Design review of the part built by this model. Coordinates are the model's own, in mm. Face numbers are marked on the shaded views. A direction names the side the tool comes from. Round coordinates to 2 decimals unless told otherwise and drop trailing zeros. Order: outer loops, then holes, each group sorted by start corner. A loop starts at its lowest first (then second) coordinate and runs counter-clockwise, first axis right, second up.
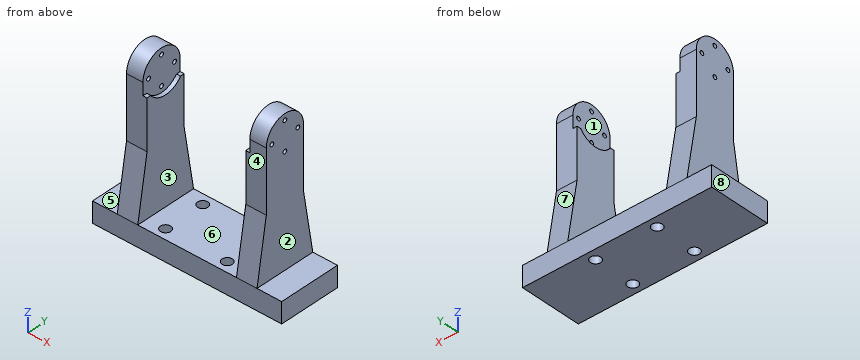
from build123d import *

# Parameters (mm, degrees)
SKETCH1_W           = 92
SKETCH1_H           = 30
BOSS_EXTRUDE1_DEPTH = 10
BOSS_EXTRUDE2_START = -12
BOSS_EXTRUDE2_DEPTH = 10
SKETCH3_R           = 1
CUT_EXTRUDE1_DEPTH  = 10
CUT_EXTRUDE2_DEPTH  = 2
SKETCH7_R           = 2.5
CUT_EXTRUDE3_DEPTH  = 10


with BuildPart() as part:
    # Sketch1 → Boss-Extrude1 (new body)
    with BuildSketch(Plane.XY):
        Rectangle(SKETCH1_W, SKETCH1_H)
    extrude(amount=BOSS_EXTRUDE1_DEPTH)

    # Sketch2 → Boss-Extrude2 (add)
    with BuildSketch(Plane(origin=(46, 0, 0), x_dir=(0, 0, -1), z_dir=(1, 0, 0)).offset(BOSS_EXTRUDE2_START)):
        with BuildLine():
            Line((-10, -15), (-10, 15))
            Line((-10, 15), (-40, 10))
            Line((-40, 10), (-70, 10))
            ThreePointArc((-70, 10), (-62.928932188, 7.071067812), (-60, 0))
            ThreePointArc((-60, 0), (-62.928932188, -7.071067812), (-70, -10))
            Line((-70, -10), (-40, -10))
            Line((-40, -10), (-10, -15))
        make_face()
        with BuildLine():
            ThreePointArc((-60, 0), (-62.928932188, 7.071067812), (-70, 10))
            Line((-70, 10), (-70, -10))
            ThreePointArc((-70, -10), (-62.928932188, -7.071067812), (-60, 0))
        make_face()
        with BuildLine():
            Line((-70, -10), (-70, 10))
            ThreePointArc((-70, 10), (-80, 0), (-70, -10))
        make_face()
    boss_extrude2 = extrude(amount=-BOSS_EXTRUDE2_DEPTH)

    # Sketch3 → Cut-Extrude1 (cut)
    with BuildSketch(Plane(origin=(34, 0, 0), x_dir=(0, 0, -1), z_dir=(1, 0, 0))):
        with Locations((-70, 7)):
            Circle(SKETCH3_R)
        with Locations((-63, 0)):
            Circle(SKETCH3_R)
        with Locations((-70, -7)):
            Circle(SKETCH3_R)
        with Locations((-77, 0)):
            Circle(SKETCH3_R)
    cut_extrude1 = extrude(amount=-CUT_EXTRUDE1_DEPTH, mode=Mode.SUBTRACT)

    # Mirror1: Boss-Extrude2, Cut-Extrude1 across plane
    add(boss_extrude2.mirror(Plane(origin=(0, 0, 0), x_dir=(0, 0, 1), z_dir=(1, 0, 0))))
    add(cut_extrude1.mirror(Plane(origin=(0, 0, 0), x_dir=(0, 0, 1), z_dir=(1, 0, 0))), mode=Mode.SUBTRACT)

    # Sketch6 → Cut-Extrude2 (cut)
    with BuildSketch(Plane.ZY.offset(-24)):
        with BuildLine():
            Line((70, 10), (64, 10))
            Line((64, 10), (64, 8))
            ThreePointArc((64, 8), (60, 0), (64, -8))
            Line((64, -8), (64, -10))
            Line((64, -10), (70, -10))
            ThreePointArc((70, -10), (80, 0), (70, 10))
        make_face()
    cut_extrude2 = extrude(amount=-CUT_EXTRUDE2_DEPTH, mode=Mode.SUBTRACT)

    # Mirror2: Cut-Extrude2 across plane
    add(cut_extrude2.mirror(Plane(origin=(0, 0, 0), x_dir=(0, 0, 1), z_dir=(1, 0, 0))), mode=Mode.SUBTRACT)

    # Sketch7 → Cut-Extrude3 (cut)
    with BuildSketch(Plane.XY.offset(10)):
        with Locations((-15, 10)):
            Circle(SKETCH7_R)
        with Locations((15, 10)):
            Circle(SKETCH7_R)
        with Locations((-15, -10)):
            Circle(SKETCH7_R)
        with Locations((15, -10)):
            Circle(SKETCH7_R)
    extrude(amount=-CUT_EXTRUDE3_DEPTH, mode=Mode.SUBTRACT)


solid = part.part
1) Take a section at A-A on z = 44.5. Give the boundary of the cut face in (x, y).
Results:
outline: (-34, -10) - (-24, -10) - (-24, 10) - (-34, 10) - close; (24, -10) - (34, -10) - (34, 10) - (24, 10) - close
2) Clearance check with flat-ended pins moving along their axes: P1, Ø15, axis at y = -6.5, z = 58.5, coming from the +X side; P2, Ø0.6, axis at x = -24.5, y = 9, coming from the +Z side; P3, Ø16, axis at y = -4.5, z = 68.5, coming from the -X side. State where each tip first meets the part, or that it passes through.
Results:
P1: stops at x = 34
P2: stops at z = 64
P3: stops at x = -34
3) Take a section at D-D on y = 4.75. Give the boundary of the cut face in (x, z).
Results:
outline: (-46, 0) - (46, 0) - (46, 10) - (34, 10) - (34, 78.8) - (26, 78.8) - (26, 61.2) - (24, 61.2) - (24, 10) - (-24, 10) - (-24, 61.2) - (-26, 61.2) - (-26, 78.8) - (-34, 78.8) - (-34, 10) - (-46, 10) - close
4) To check wall thickness, follow line 1 along Y through (x, z) = (-32, 70); line 2 along Z through (x, y) = (-30.75, 0); line 3 along Y through (x, z) = (15, 3.75). State the ranges of each line that lie inside material, in increasing order.
Results:
line 1: y = -10 to -8, -6 to 6, 8 to 10
line 2: z = 0 to 62, 64 to 76, 78 to 80
line 3: y = -15 to -12.5, -7.5 to 7.5, 12.5 to 15
5) The part is to be moulded in two halves that separate along X. For the marked faces 6, 7 and 8, say which applies: released by +X, released by -X, zero draft, split by the parting line, or undercut.
Results:
face 6: undercut
face 7: zero draft
face 8: released by -X
6) Take a section at B-B on x = 15. Give the boundary of the cut face in (y, z).
Results:
outline: (-15, 0) - (-12.5, 0) - (-12.5, 10) - (-15, 10) - close; (-7.5, 0) - (7.5, 0) - (7.5, 10) - (-7.5, 10) - close; (12.5, 0) - (15, 0) - (15, 10) - (12.5, 10) - close
7) Take a section at C-C on x = -29.5. Give the boundary of the cut face in (y, z), plus the area to 3 significant figures.
Results:
outline: (-15, 0) - (15, 0) - (15, 10) - (10, 40) - (10, 70) arc R10 ccw to (-10, 70) - (-10, 40) - (-15, 10) - close; hole circle Ø2 at (-7, 70); hole circle Ø2 at (0, 63); hole circle Ø2 at (0, 77); hole circle Ø2 at (7, 70)
area: 1,790 mm2
8) For the marked faces 1, 2, 3, 4 and 5, list the 3-axis set-ups (+Z, -Z, +X, -X, +Y, -Y) from which the entire face can be reached by the end or side of a thin tool; tool diameter is ignored.
Results:
face 1: +Z
face 2: +Z, +X, +Y, -Y
face 3: +Z, +Y, -Y
face 4: +Z, +X, -X, -Y
face 5: +Z, -X, +Y, -Y
